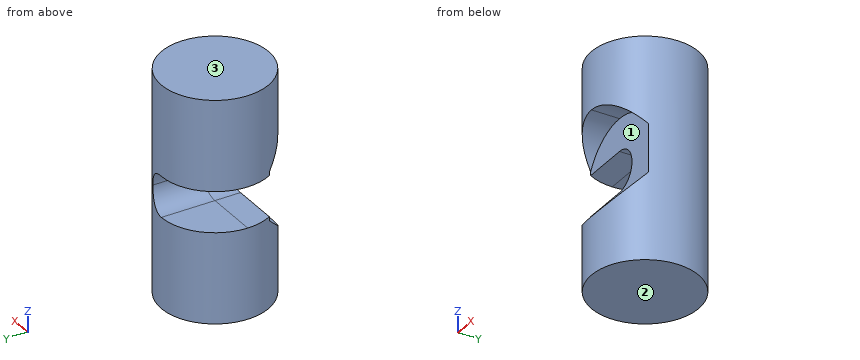
from build123d import *

# Parameters (mm, degrees)
F0_R          = 4.2
F2_DEPTH      = 8.7
F2_DEPTH_BACK = 8.7
F3_START      = 2
F3_DEPTH      = 3
F4_DEPTH      = 25
F4_DEPTH_BACK = 25


with BuildPart() as f2:
    # F0 (on Top) → F2 (new body, two sides)
    with BuildSketch(Plane.XY) as f2_sk:
        Circle(F0_R)
    extrude(amount=F2_DEPTH)
    extrude(f2_sk.sketch, amount=-F2_DEPTH_BACK)

    # F1 (on Front) → F3 (cut)
    with BuildSketch(Plane.XZ.offset(F3_START)):
        with BuildLine():
            ThreePointArc((0, -4.15), (2.9344931419, -2.9344931419), (4.15, 0))
            ThreePointArc((4.15, 0), (2.9344931419, 2.9344931419), (0, 4.15))
            ThreePointArc((0, 4.15), (-2.3002717231, 3.4541641536), (-3.8291643997, 1.6))
            Line((-3.8291643997, 1.6), (0, 1.6))
            ThreePointArc((0, 1.6), (1.1313708499, 1.1313708499), (1.6, 0))
            ThreePointArc((1.6, 0), (1.1313708499, -1.1313708499), (0, -1.6))
            Line((0, -1.6), (-3.8291643997, -1.6))
            ThreePointArc((-3.8291643997, -1.6), (-2.3002717231, -3.4541641536), (0, -4.15))
        make_face()
    extrude(amount=F3_DEPTH, mode=Mode.SUBTRACT)

    # F1 (on Front) → F4 (cut, two sides)
    with BuildSketch(Plane.XZ) as f4_sk:
        with BuildLine():
            Line((0, 1.6), (-3.8291643997, 1.6))
            ThreePointArc((-3.8291643997, 1.6), (-4.0690006303, 0.8159251624), (-4.15, 0))
            ThreePointArc((-4.15, 0), (-4.0690006303, -0.8159251624), (-3.8291643997, -1.6))
            Line((-3.8291643997, -1.6), (0, -1.6))
            ThreePointArc((0, -1.6), (-1.6, 0), (0, 1.6))
        make_face()
        with BuildLine():
            ThreePointArc((1.6, 0), (1.1313708499, 1.1313708499), (0, 1.6))
            ThreePointArc((0, 1.6), (-1.6, 0), (0, -1.6))
            ThreePointArc((0, -1.6), (1.1313708499, -1.1313708499), (1.6, 0))
        make_face()
        with BuildLine():
            Line((-4.15, -1.6), (-3.8291643997, -1.6))
            ThreePointArc((-3.8291643997, -1.6), (-4.0690006303, -0.8159251624), (-4.15, 0))
            Line((-4.15, 0), (-4.15, -1.6))
        make_face()
        with BuildLine():
            ThreePointArc((-4.15, 0), (-4.0690006303, 0.8159251624), (-3.8291643997, 1.6))
            Line((-3.8291643997, 1.6), (-4.15, 1.6))
            Line((-4.15, 1.6), (-4.15, 0))
        make_face()
        Polygon((-4.15, -1.6), (-4.15, 0), (-4.15, 1.6), (-4.2, 1.6), (-4.2, -1.6), align=None)
    extrude(amount=-F4_DEPTH, mode=Mode.SUBTRACT)
    extrude(f4_sk.sketch, amount=F4_DEPTH_BACK, mode=Mode.SUBTRACT)


solid = f2.part
Input: part model. Units: mm. Frame: model coordinates. Face numbers are marked on the shaded views. Coordinates: 2 decimals unless noted, no trailing zeros. Loops run counter-clockwise (first coordinate to the right, second up) from the corner with the lowest first, then second, coordinate; pieces in that order, holes last.
(1) Section C-C on z = -6. Return the cut outline in (x, y), then the cut area to 3 significant figures.
(2) Section D-D on x = -1.75. Return the cut outline in (y, z), then the cut area to 3 significant figures.
(3) Section B-B on x = 2.5. Return the cut outline in (y, z).
(4) Material intervals for probe 1 along Z at (x, y) = (-1.25, 3.5); probe 2 along Z at (x, y) = (0.75, 3.5); probe 3 along Y at (x, z) = (2, -4), sorted ascending.
(5) First-contact query: pin 1 Ø4 at (x, z) = (-2.5, -1.5) entering from +Y; pin 2 Ø1.5 at (y, z) = (-2, -4.5) entering from -X. Flat tips, straight axial feed; report the tip coordinate or a pass-through.
(6) Pull-direction query (Z, two-part tool) for the marked faces 1, 2 and 3; classes: released by +Z, released by -Z, zero draft, split by the parting line, or undercut.
(7) Section A-A on x = 0.75. Return the cut outline in (y, z).
Data:
1. outline: circle Ø8.4 at (0, 0)
1. area: 55.4 mm2
2. outline: (-3.82, -8.7) - (3.82, -8.7) - (3.82, -1.6) - (-2, -1.6) - (-2, -3.76) - (-3.82, -3.76) - close; (-3.82, 3.76) - (-2, 3.76) - (-2, 1.6) - (3.82, 1.6) - (3.82, 8.7) - (-3.82, 8.7) - close
2. area: 101 mm2
3. outline: (-3.37, -8.7) - (3.37, -8.7) - (3.37, 8.7) - (-3.37, 8.7) - (-3.37, 3.31) - (-2, 3.31) - (-2, -3.31) - (-3.37, -3.31) - close
4. probe 1: z = -8.7 to -1.6, 1.6 to 8.7
4. probe 2: z = -8.7 to -1.41, 1.41 to 8.7
4. probe 3: y = -3.69 to 3.69
5. pin 1: stops at y = 4.17
5. pin 2: stops at x = -4.01
6. face 1: undercut
6. face 2: released by -Z
6. face 3: released by +Z
7. outline: (-4.13, -8.7) - (4.13, -8.7) - (4.13, -1.41) - (-2, -1.41) - (-2, -4.08) - (-4.13, -4.08) - close; (-4.13, 4.08) - (-2, 4.08) - (-2, 1.41) - (4.13, 1.41) - (4.13, 8.7) - (-4.13, 8.7) - close
